from build123d import *

# Parameters (mm, degrees)
F0_R     = 1.5
F1_DEPTH = 12.7
F2_W     = 408
F2_H     = 258
F2_W_2   = 59
F2_H_2   = 132
F3_DEPTH = 1


with BuildPart() as f1:
    # F0 (on Top) → F1 (new body)
    with BuildSketch(Plane.XY):
        Polygon((103.953788, 154.93784), (-336.046212, 154.93784), (-336.046212, 59.93784), (-356.046212, 59.93784), (-356.046212, -40.06216), (-336.046212, -40.06216), (-336.046212, -135.06216), (103.953788, -135.06216), (103.953788, -40.06216), (123.953788, -40.06216), (123.953788, 59.93784), (103.953788, 59.93784), align=None)
        with Locations((-329.696212, -120.06216)):
            Circle(F0_R, mode=Mode.SUBTRACT)
        with Locations((-306.046212, -128.71216)):
            Circle(F0_R, mode=Mode.SUBTRACT)
        with Locations((-329.701892, -100.062161)):
            Circle(F0_R, mode=Mode.SUBTRACT)
        with Locations((-286.046212, -128.71216)):
            Circle(F0_R, mode=Mode.SUBTRACT)
        with Locations((-266.046212, -128.71216)):
            Circle(F0_R, mode=Mode.SUBTRACT)
        with Locations((-246.046212, -128.71216)):
            Circle(F0_R, mode=Mode.SUBTRACT)
        with Locations((-329.707572, -80.062162)):
            Circle(F0_R, mode=Mode.SUBTRACT)
        with Locations((-226.046212, -128.71216)):
            Circle(F0_R, mode=Mode.SUBTRACT)
        with Locations((-206.046212, -128.71216)):
            Circle(F0_R, mode=Mode.SUBTRACT)
        with Locations((-186.046212, -128.71216)):
            Circle(F0_R, mode=Mode.SUBTRACT)
        with Locations((-166.046212, -128.71216)):
            Circle(F0_R, mode=Mode.SUBTRACT)
        with Locations((-146.046212, -128.71216)):
            Circle(F0_R, mode=Mode.SUBTRACT)
        with Locations((-126.046212, -128.71216)):
            Circle(F0_R, mode=Mode.SUBTRACT)
        with Locations((-329.713253, -60.062163)):
            Circle(F0_R, mode=Mode.SUBTRACT)
        with Locations((-329.718933, -40.062164)):
            Circle(F0_R, mode=Mode.SUBTRACT)
        with Locations((-106.046212, -128.71216)):
            Circle(F0_R, mode=Mode.SUBTRACT)
        with Locations((-86.046212, -128.71216)):
            Circle(F0_R, mode=Mode.SUBTRACT)
        with Locations((-66.046212, -128.71216)):
            Circle(F0_R, mode=Mode.SUBTRACT)
        with Locations((-46.046212, -128.71216)):
            Circle(F0_R, mode=Mode.SUBTRACT)
        with Locations((-26.046212, -128.71216)):
            Circle(F0_R, mode=Mode.SUBTRACT)
        with Locations((-6.046212, -128.71216)):
            Circle(F0_R, mode=Mode.SUBTRACT)
        with Locations((13.953788, -128.71216)):
            Circle(F0_R, mode=Mode.SUBTRACT)
        with Locations((33.953788, -128.71216)):
            Circle(F0_R, mode=Mode.SUBTRACT)
        with Locations((53.953788, -128.71216)):
            Circle(F0_R, mode=Mode.SUBTRACT)
        with Locations((73.953788, -128.71216)):
            Circle(F0_R, mode=Mode.SUBTRACT)
        with Locations((97.603788, -120.06216)):
            Circle(F0_R, mode=Mode.SUBTRACT)
        with Locations((97.609468, -100.062161)):
            Circle(F0_R, mode=Mode.SUBTRACT)
        with Locations((97.615149, -80.062162)):
            Circle(F0_R, mode=Mode.SUBTRACT)
        with Locations((97.620829, -60.062163)):
            Circle(F0_R, mode=Mode.SUBTRACT)
        with BuildLine():
            Line((-331.046212, 47.23784), (-331.046212, -27.36216))
            Line((-331.046212, -27.36216), (-338.346212, -27.36216))
            ThreePointArc((-338.346212, -27.36216), (-347.326468, -23.642417), (-351.046212, -14.66216))
            Line((-351.046212, -14.66216), (-351.046212, 34.53784))
            ThreePointArc((-351.046212, 34.53784), (-347.326468, 43.518096), (-338.346212, 47.23784))
            Line((-338.346212, 47.23784), (-331.046212, 47.23784))
        make_face(mode=Mode.SUBTRACT)
        with Locations((-329.713253, 79.937842)):
            Circle(F0_R, mode=Mode.SUBTRACT)
        with Locations((-329.707572, 99.937841)):
            Circle(F0_R, mode=Mode.SUBTRACT)
        with Locations((-329.701892, 119.93784)):
            Circle(F0_R, mode=Mode.SUBTRACT)
        with Locations((-329.696212, 139.93784)):
            Circle(F0_R, mode=Mode.SUBTRACT)
        with Locations((-306.046212, 148.58784)):
            Circle(F0_R, mode=Mode.SUBTRACT)
        with Locations((-286.046212, 148.58784)):
            Circle(F0_R, mode=Mode.SUBTRACT)
        with Locations((-266.046212, 148.58784)):
            Circle(F0_R, mode=Mode.SUBTRACT)
        with Locations((-246.046212, 148.58784)):
            Circle(F0_R, mode=Mode.SUBTRACT)
        with Locations((-226.046212, 148.58784)):
            Circle(F0_R, mode=Mode.SUBTRACT)
        with Locations((-206.046212, 148.58784)):
            Circle(F0_R, mode=Mode.SUBTRACT)
        with Locations((-186.046212, 148.58784)):
            Circle(F0_R, mode=Mode.SUBTRACT)
        with Locations((-166.046212, 148.58784)):
            Circle(F0_R, mode=Mode.SUBTRACT)
        with Locations((-146.046212, 148.58784)):
            Circle(F0_R, mode=Mode.SUBTRACT)
        with Locations((-126.046212, 148.58784)):
            Circle(F0_R, mode=Mode.SUBTRACT)
        with BuildLine():
            Line((106.253788, -27.36216), (98.953788, -27.36216))
            Line((98.953788, -27.36216), (98.953788, 47.23784))
            Line((98.953788, 47.23784), (106.253788, 47.23784))
            ThreePointArc((106.253788, 47.23784), (115.234044, 43.518096), (118.953788, 34.53784))
            Line((118.953788, 34.53784), (118.953788, -14.66216))
            ThreePointArc((118.953788, -14.66216), (115.234044, -23.642417), (106.253788, -27.36216))
        make_face(mode=Mode.SUBTRACT)
        with Locations((97.620829, 79.937842)):
            Circle(F0_R, mode=Mode.SUBTRACT)
        with Locations((-106.046212, 148.58784)):
            Circle(F0_R, mode=Mode.SUBTRACT)
        with Locations((-86.046212, 148.58784)):
            Circle(F0_R, mode=Mode.SUBTRACT)
        with Locations((-66.046212, 148.58784)):
            Circle(F0_R, mode=Mode.SUBTRACT)
        with Locations((-46.046212, 148.58784)):
            Circle(F0_R, mode=Mode.SUBTRACT)
        with Locations((-26.046212, 148.58784)):
            Circle(F0_R, mode=Mode.SUBTRACT)
        with Locations((-6.046212, 148.58784)):
            Circle(F0_R, mode=Mode.SUBTRACT)
        with Locations((97.615149, 99.937841)):
            Circle(F0_R, mode=Mode.SUBTRACT)
        with Locations((13.953788, 148.58784)):
            Circle(F0_R, mode=Mode.SUBTRACT)
        with Locations((33.953788, 148.58784)):
            Circle(F0_R, mode=Mode.SUBTRACT)
        with Locations((53.953788, 148.58784)):
            Circle(F0_R, mode=Mode.SUBTRACT)
        with Locations((97.609468, 119.93784)):
            Circle(F0_R, mode=Mode.SUBTRACT)
        with Locations((73.953788, 148.58784)):
            Circle(F0_R, mode=Mode.SUBTRACT)
        with Locations((97.603788, 139.93784)):
            Circle(F0_R, mode=Mode.SUBTRACT)
    extrude(amount=F1_DEPTH)

    # F2 (on face) → F3 (join)
    with BuildSketch(Plane.XY.offset(12.7)):
        with Locations((-116.046212, 9.93784)):
            Rectangle(F2_W, F2_H)
        with Locations((-288.546212, 9.93784)):
            Rectangle(F2_W_2, F2_H_2, mode=Mode.SUBTRACT)
        with BuildLine():
            Line((-318.046212, 76.93784), (-318.046212, 136.93784))
            Line((-318.046212, 136.93784), (-116.546212, 136.93784))
            Line((-116.546212, 136.93784), (-116.546212, 54.935062))
            ThreePointArc((-116.546212, 54.935062), (-161.046212, 9.93784), (-116.546212, -35.059383))
            Line((-116.546212, -35.059383), (-116.546212, -117.06216))
            Line((-116.546212, -117.06216), (-318.046212, -117.06216))
            Line((-318.046212, -117.06216), (-318.046212, -57.06216))
            Line((-318.046212, -57.06216), (-258.046212, -57.06216))
            Line((-258.046212, -57.06216), (-258.046212, 76.93784))
            Line((-258.046212, 76.93784), (-318.046212, 76.93784))
        make_face(mode=Mode.SUBTRACT)
        with BuildLine():
            ThreePointArc((-116.546212, -34.559351), (-160.546212, 9.93784), (-116.546212, 54.435031))
            Line((-116.546212, 54.435031), (-116.546212, -34.559351))
        make_face(mode=Mode.SUBTRACT)
        with BuildLine():
            Line((-115.546212, -34.559351), (-115.546212, 54.435031))
            ThreePointArc((-115.546212, 54.435031), (-71.546212, 9.93784), (-115.546212, -34.559351))
        make_face(mode=Mode.SUBTRACT)
        with BuildLine():
            Line((-115.546212, 136.93784), (85.953788, 136.93784))
            Line((85.953788, 136.93784), (85.953788, 76.93784))
            Line((85.953788, 76.93784), (25.953788, 76.93784))
            Line((25.953788, 76.93784), (25.953788, -57.06216))
            Line((25.953788, -57.06216), (85.953788, -57.06216))
            Line((85.953788, -57.06216), (85.953788, -117.06216))
            Line((85.953788, -117.06216), (-115.546212, -117.06216))
            Line((-115.546212, -117.06216), (-115.546212, -35.059383))
            ThreePointArc((-115.546212, -35.059383), (-71.046212, 9.93784), (-115.546212, 54.935062))
            Line((-115.546212, 54.935062), (-115.546212, 136.93784))
        make_face(mode=Mode.SUBTRACT)
        with Locations((56.453788, 9.93784)):
            Rectangle(F2_W_2, F2_H_2, mode=Mode.SUBTRACT)
    extrude(amount=F3_DEPTH)


solid = f1.part
The listing builds one solid part. Answer for the finished solid, in the listing's coordinates (mm). A direction names the side the tool comes from. Give positions to 0.01 mm unless a question says otherwise; leave off trailing zeros. Order: outer loops, then holes, each group sorted by start corner. A loop starts at its lowest first (then second) coordinate and runs counter-clockwise, first axis right, second up. Notation, with made-up numbers: (35.25, 7.25) - (80.25, 7.25) arc R18 ccw to (80.25, 18.25) - close; hole circle Ø9 at (47, 28.25). An arc over 180 degrees is marked (long way). One line per item, written item: value. Start each with the question number.
1) A cutting plane is placed at C-C on y = -4. State how many separate pieces and enclosed holes the cut face has, then the cut area to 3 significant figures.
2) The mould has two halves that part along X. Classify faces 1 (the face through (103.954, 107, 6)), 2 (the face through (-16, 12, 12.7)), 3 (the face through (-336.046, -87, 6)): released by +X, released by -X, zero draft, split by the parting line, or undercut.
3) A cutting plane is placed at B-B on x = -236.5. Give the vertices of the cut face in (y, z).
4) A cutting plane is placed at A-A on y = 132. Give the vertices of the cut face in (x, z).
5) A tool of negligible diameter and unlimited length cuts with its end or side. For faces 4 (the face through (-134, 11, 12.7)), 5 (the face through (114, -40.062, 6)), 6 (the face through (-113, 154.938, 6)), 7 (the face through (115.13, 43.62, 6.26)), 8 (the face through (-346, 59.938, 6)), from which of +Z, -Z, +X, -X, +Y, -Y can it reach the whole face along a straight path? Write none if from no direction.
6) Find the intervals of material crossed by L1, parallel to X at y = 94, z = 13; L2, parallel to Y at x = -126.5, z = 2.75; L3, parallel to Z at x = 82, y = 70, in increasing order.
7) Given pin 1 Ø1.5 at (y, z) = (108, 11) entering from -X; pin 2 Ø1.1 at (y, z) = (-82.5, 13.5) entering from -X; pin 3 Ø0.5 at (x, z) = (60.5, 13.5) entering from -Y, each flat-ended and moving along its own axis, determine where each tip first touches the part or whether it passes through.
Answer sheet:
1. separate pieces: 3
1. enclosed holes: 0
1. area: 5,600 mm2
2. face 1: released by +X
2. face 2: undercut
2. face 3: released by -X
3. outline: (-135.06, 0) - (154.94, 0) - (154.94, 12.7) - (138.94, 12.7) - (138.94, 13.7) - (136.94, 13.7) - (136.94, 12.7) - (-117.06, 12.7) - (-117.06, 13.7) - (-119.06, 13.7) - (-119.06, 12.7) - (-135.06, 12.7) - close
4. outline: (-336.05, 0) - (103.95, 0) - (103.95, 12.7) - (87.95, 12.7) - (87.95, 13.7) - (85.95, 13.7) - (85.95, 12.7) - (-115.55, 12.7) - (-115.55, 13.7) - (-116.55, 13.7) - (-116.55, 12.7) - (-318.05, 12.7) - (-318.05, 13.7) - (-320.05, 13.7) - (-320.05, 12.7) - (-336.05, 12.7) - close
5. face 4: +Z
5. face 5: +Z, -Z, +X, -Y
5. face 6: +Z, -Z, +X, -X, +Y
5. face 7: +Z, -Z
5. face 8: +Z, -Z, -X, +Y
6. L1: x = -320.05 to -318.05, -116.55 to -115.55, 85.95 to 87.95
6. L2: y = -135.06 to -130.14, -127.28 to 147.16, 150.02 to 154.94
6. L3: z = 0 to 12.7
7. pin 1: stops at x = -336.05
7. pin 2: stops at x = -320.05
7. pin 3: stops at y = -119.06
